from build123d import *

# Parameters (mm, degrees)
F0_R     = 4
F0_R_2   = 56
F1_DEPTH = 13.5


with BuildPart() as f1:
    # F0 (on Front) → F1 (new body, symmetric)
    with BuildSketch(Plane.XZ):
        with BuildLine():
            ThreePointArc((-90, -150), (-81.213203, -171.213203), (-60, -180))
            Line((-60, -180), (60, -180))
            ThreePointArc((60, -180), (81.213203, -171.213203), (90, -150))
            Line((90, -150), (90, 27))
            Line((90, 27), (-90, 27))
            Line((-90, 27), (-90, -150))
        make_face()
        with Locations((-65, -90)):
            Circle(F0_R, mode=Mode.SUBTRACT)
        with Locations((0, -155)):
            Circle(F0_R, mode=Mode.SUBTRACT)
        with Locations((0, -90)):
            Circle(F0_R_2, mode=Mode.SUBTRACT)
        with Locations((65, -90)):
            Circle(F0_R, mode=Mode.SUBTRACT)
        with Locations((-75, 13.5)):
            Circle(F0_R, mode=Mode.SUBTRACT)
        with Locations((-25, 13.5)):
            Circle(F0_R, mode=Mode.SUBTRACT)
        with Locations((0, -25)):
            Circle(F0_R, mode=Mode.SUBTRACT)
        with Locations((25, 13.5)):
            Circle(F0_R, mode=Mode.SUBTRACT)
        with Locations((75, 13.5)):
            Circle(F0_R, mode=Mode.SUBTRACT)
    extrude(amount=F1_DEPTH, both=True)


solid = f1.part
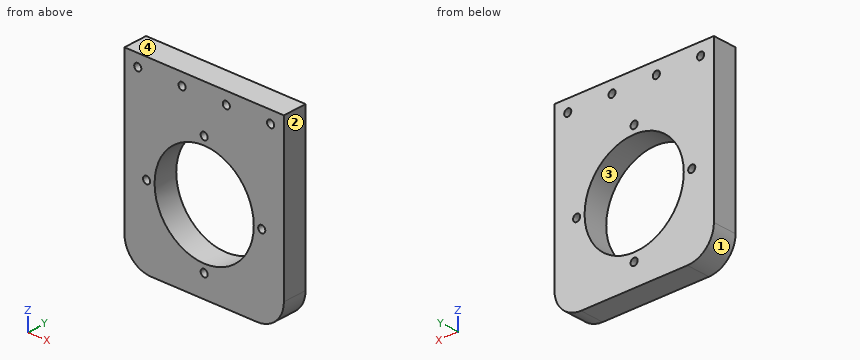
The listing builds one solid part. Answer for the finished solid, in the listing's coordinates (mm). Face numbers are marked on the shaded views. Give positions to 0.01 mm unless a question says otherwise; leave off trailing zeros. Write each loop counter-clockwise with the first axis right and the second up, starting at its lowest first coordinate (ties: lowest second). Pieces come first, ordered by that corner, then holes. Notation, with made-up numbers: (-27.75, -3.5) - (-19.75, -3.5) arc R30 ccw to (-19.75, 27.5) - close; hole circle Ø4 at (34, 85). An arc over 180 degrees is marked (long way). One line per question, with ' | ' between items. Start each with the question number.
1. Given P1, Ø6.5, axis at x = -25, z = 13.5, coming from the -Y side, flat-ended and moving along its own axis, determine where the tip first touches the part or whether it passes through.
2. Determine the mould class of the marked faces 1, 2, 3 and 4 for opening direction Z: +Z half, -Z half, draft (parallel to the pull), parting line (faces both ways), or undercut.
3. Section B-B, the plane y = 1 is taken. Count the separate pieces of the cut face and the enclosed holes in it, then the cut area to 3 significant figures.
4. Straight lines are drawn through the part: line 1 (Z direction, x = 0, y = -1.25); line 2 (Z direction, x = -24.5, y = -0.5); line 3 (Z direction, x = -25, y = -0.25). For each, find the intervals that lie inside material, in ascending order.
5. Section C-C, the plane z = -90 is taken. Determine the outline of the cut face in (x, y).
6. Section A-A, the plane x = 0 is taken. Determine the outline of the cut face in (y, z).
7. Section D-D, the plane x = 65 is taken. Determine the outline of the cut face in (y, z).
Result:
1) P1: passes through
2) face 1: -Z half | face 2: draft | face 3: undercut | face 4: +Z half
3) separate pieces: 1 | enclosed holes: 9 | area: 26,600 mm2
4) line 1: z = -180 to -159, -151 to -146, -34 to -29, -21 to 27 | line 2: z = -180 to -140.36, -39.64 to 9.53, 17.47 to 27 | line 3: z = -180 to -140.11, -39.89 to 9.5, 17.5 to 27
5) outline: (-90, -13.5) - (-69, -13.5) - (-69, 13.5) - (-90, 13.5) - close; (-61, -13.5) - (-56, -13.5) - (-56, 13.5) - (-61, 13.5) - close; (56, -13.5) - (61, -13.5) - (61, 13.5) - (56, 13.5) - close; (69, -13.5) - (90, -13.5) - (90, 13.5) - (69, 13.5) - close
6) outline: (-13.5, -180) - (13.5, -180) - (13.5, -159) - (-13.5, -159) - close; (-13.5, -151) - (13.5, -151) - (13.5, -146) - (-13.5, -146) - close; (-13.5, -34) - (13.5, -34) - (13.5, -29) - (-13.5, -29) - close; (-13.5, -21) - (13.5, -21) - (13.5, 27) - (-13.5, 27) - close
7) outline: (-13.5, -179.58) - (13.5, -179.58) - (13.5, -94) - (-13.5, -94) - close; (-13.5, -86) - (13.5, -86) - (13.5, 27) - (-13.5, 27) - close
